Geometry: final body of the model. Coordinates: model frame, mm. Face numbers are marked on the shaded views. A direction names the side the tool comes from. Give positions to 0.01 mm unless a question says otherwise; leave off trailing zeros. Order: outer loops, then holes, each group sorted by start corner. A loop starts at its lowest first (then second) coordinate and runs counter-clockwise, first axis right, second up. Notation, with made-up numbers: (-18, 87.5) - (8, 87.5) arc R35 ccw to (8, 124.5) - close; hole circle Ø10 at (-37.5, 47.25). An arc over 180 degrees is marked (long way). Use one line per item in the form item = value.
from build123d import *

# Parameters (mm, degrees)
SKETCH1_W           = 76.947055408
SKETCH1_H           = 56
SKETCH1_R           = 1.1
SKETCH1_W_2         = 9
SKETCH1_H_2         = 34
BOSS_EXTRUDE1_DEPTH = 4
SKETCH6_W           = 4
SKETCH6_H           = 30
BOSS_EXTRUDE5_DEPTH = 20
SKETCH7_W           = 70
SKETCH7_H           = 4
BOSS_EXTRUDE6_DEPTH = 20
SKETCH8_R           = 4.55
CUT_EXTRUDE2_DEPTH  = 4
SKETCH9_R           = 7.55
CUT_EXTRUDE3_DEPTH  = 2
SKETCH10_R          = 2
CUT_EXTRUDE4_DEPTH  = 1.5
FILLET4_R           = 1


with BuildPart() as part:
    # Sketch1 → Boss-Extrude1 (new body)
    with BuildSketch(Plane(origin=(0, 0, 0), x_dir=(1, 0, 0), z_dir=(0, 1, 0))):
        Rectangle(SKETCH1_W, SKETCH1_H)
        with Locations((-31.5, 20.5)):
            Circle(SKETCH1_R, mode=Mode.SUBTRACT)
        with Locations((-31.5, -20.5)):
            Circle(SKETCH1_R, mode=Mode.SUBTRACT)
        with Locations((31.5, -20.5)):
            Circle(SKETCH1_R, mode=Mode.SUBTRACT)
        with Locations((31.5, 20.5)):
            Circle(SKETCH1_R, mode=Mode.SUBTRACT)
        with Locations((-31.5, 0)):
            Rectangle(SKETCH1_W_2, SKETCH1_H_2, mode=Mode.SUBTRACT)
    extrude(amount=BOSS_EXTRUDE1_DEPTH)

    # Sketch6 → Boss-Extrude5 (add)
    with BuildSketch(Plane(origin=(0, 4, 0), x_dir=(1, 0, 0), z_dir=(0, 1, 0))):
        with Locations((-17.5, 0)):
            Rectangle(SKETCH6_W, SKETCH6_H)
    boss_extrude5 = extrude(amount=BOSS_EXTRUDE5_DEPTH)

    # Sketch7 → Boss-Extrude6 (add)
    with BuildSketch(Plane.ZY.offset(19.5)):
        with Locations((0, 22)):
            Rectangle(SKETCH7_W, SKETCH7_H)
    boss_extrude6 = extrude(amount=BOSS_EXTRUDE6_DEPTH)

    # Sketch8 → Cut-Extrude2 (cut)
    with BuildSketch(Plane(origin=(0, 24, 0), x_dir=(1, 0, 0), z_dir=(0, 1, 0))):
        with Locations((-29.5, 25)):
            Circle(SKETCH8_R)
        with Locations((-29.5, -25)):
            Circle(SKETCH8_R)
    cut_extrude2 = extrude(amount=-CUT_EXTRUDE2_DEPTH, mode=Mode.SUBTRACT)

    # Sketch9 → Cut-Extrude3 (cut)
    with BuildSketch(Plane(origin=(0, 24, 0), x_dir=(1, 0, 0), z_dir=(0, 1, 0))):
        with Locations((-29.5, 25)):
            Circle(SKETCH9_R)
        with Locations((-29.5, -25)):
            Circle(SKETCH9_R)
    cut_extrude3 = extrude(amount=-CUT_EXTRUDE3_DEPTH, mode=Mode.SUBTRACT)

    # Mirror2: Boss-Extrude5, Boss-Extrude6, Cut-Extrude2, Cut-Extrude3 across plane
    add(boss_extrude5.mirror(Plane(origin=(0, 0, 0), x_dir=(0, 0, 1), z_dir=(1, 0, 0))))
    add(boss_extrude6.mirror(Plane(origin=(0, 0, 0), x_dir=(0, 0, 1), z_dir=(1, 0, 0))))
    add(cut_extrude2.mirror(Plane(origin=(0, 0, 0), x_dir=(0, 0, 1), z_dir=(1, 0, 0))), mode=Mode.SUBTRACT)
    add(cut_extrude3.mirror(Plane(origin=(0, 0, 0), x_dir=(0, 0, 1), z_dir=(1, 0, 0))), mode=Mode.SUBTRACT)

    # Sketch10 → Cut-Extrude4 (cut)
    with BuildSketch(Plane(origin=(0, 4, 0), x_dir=(1, 0, 0), z_dir=(0, 1, 0))):
        with Locations((-31.5, -20.5)):
            Circle(SKETCH10_R)
        with Locations((-31.5, 20.5)):
            Circle(SKETCH10_R)
        with Locations((31.5, 20.5)):
            Circle(SKETCH10_R)
        with Locations((31.5, -20.5)):
            Circle(SKETCH10_R)
    extrude(amount=-CUT_EXTRUDE4_DEPTH, mode=Mode.SUBTRACT)

    # Fillet4
    fillet4_edges = [part.edges().sort_by_distance(p)[0] for p in [
        (-38.473527704, 4, 0),
        (17.5, 4, 15),
        (19.5, 22, 35),
        (39.5, 22, 35),
        (29.5, 24, 35),
        (39.5, 20, 0),
        (29.5, 20, 35),
        (39.5, 22, -35),
        (29.5, 20, -35),
        (39.5, 24, 0),
        (29.5, 24, -35),
        (19.5, 22, -35),
        (0, 4, 28),
        (38.473527704, 4, 0),
        (0, 0, 28),
        (-15.5, 4, 0),
        (-15.5, 14, 15),
        (-17.5, 4, -15),
        (-15.5, 14, -15),
        (-17.5, 4, 15),
        (-15.5, 24, 0),
        (-38.473527704, 0, 0),
        (0, 0, -28),
        (38.473527704, 0, 0),
        (-19.5, 22, 35),
        (-29.5, 20, 35),
        (-29.5, 24, 35),
        (-19.5, 22, -35),
        (-29.5, 24, -35),
        (-29.5, 20, -35),
        (-39.5, 22, 35),
        (-39.5, 24, 0),
        (-39.5, 22, -35),
        (-39.5, 20, 0),
        (0, 4, -28),
        (38.473527704, 2, 28),
        (-38.473527704, 2, 28),
        (-38.473527704, 2, -28),
        (38.473527704, 2, -28),
        (15.5, 24, 0),
        (15.5, 14, -15),
        (15.5, 14, 15),
        (15.5, 4, 0),
        (17.5, 4, -15),
    ]]
    fillet(fillet4_edges, radius=FILLET4_R)


solid = part.part
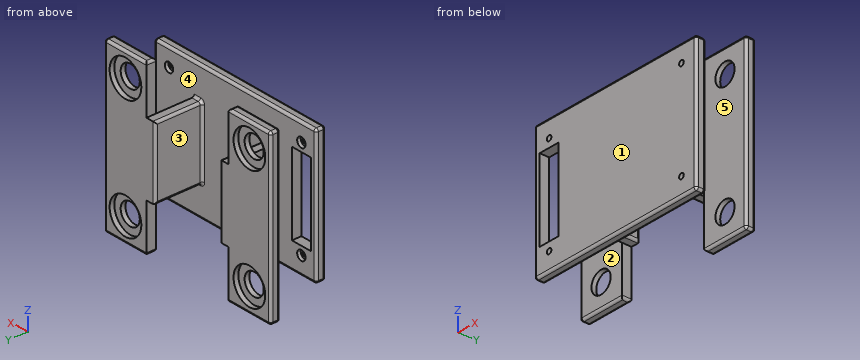
(1) Pull-direction query (X, two-part tool) for the marked faces 4 and 5; classes: released by +X, released by -X, zero draft, split by the parting line, or undercut.
Computed values:
face_4 = undercut
face_5 = zero draft
(2) Reachability of the marked faces 1, 2 and 3 from +Z, -Z, +X, -X, +Y, -Y: full face, straight path, thin tool, end or side. Return the list, or none.
Computed values:
face_1 = +Z, -Z, +X, -X, -Y
face_2 = +Z, -Z, -X
face_3 = +Z, -Z, +Y
(3) Cut plane C-C on x = -13.5. Output: boundary loops of the cut face in (y, z).
Computed values:
outline = (0, -27) arc R1 ccw to (1, -28) - (3, -28) arc R1 ccw to (4, -27) - (4, 27) arc R1 ccw to (3, 28) - (1, 28) arc R1 ccw to (0, 27) - close
(4) Contact query for flat-ended pins moving along their axis: pin 1 Ø1.2 at (y, z) = (1, -3) entering from -X; pin 2 Ø0.6 at (y, z) = (1.5, -1) entering from +X; pin 3 Ø12 at (y, z) = (9.5, 22.5) entering from -X. Output: stop coordinate, or through.
Computed values:
pin_1 = -38.47
pin_2 = 38.47
pin_3 = -38.34
(5) Cut plane B-B on y = 8.5. Output: boundary loops of the cut face in (x, z), plus the area to 3 significant figures.
Computed values:
outline = (-19.5, -15) - (-16.5, -15) arc R1 ccw to (-15.5, -14) - (-15.5, 14) arc R1 ccw to (-16.5, 15) - (-19.5, 15) - close; (15.5, -14) arc R1 ccw to (16.5, -15) - (19.5, -15) - (19.5, 15) - (16.5, 15) arc R1 ccw to (15.5, 14) - close
area = 239 mm²
(6) Ray query, line 1 along X through (y, z) = (22.95, 25); line 2 along Z through (x, y) = (-29.5, 20.95); line 3 along Z through (x, y) = (-31.5, 1.3). Return the intervals inside material, ascending.
Computed values:
line_1 = -39.5 to -37.05, -21.95 to -19.5, 19.5 to 21.95, 37.05 to 39.5
line_2 = -35 to -29.55, -20.45 to 20.45, 29.55 to 35
line_3 = -28 to -21.6, -19.4 to -17, 17 to 19.4, 21.6 to 28
(7) Cut plane D-D on z = -25. Give the number of separate pieces and of enclosed holes in the cut face, plus the area to 3 significant figures.
Computed values:
separate_pieces = 5
enclosed_holes = 0
area = 369 mm²
